Part model, mm, in its own coordinate system. A direction names the side the tool comes from. Give positions to 0.01 mm unless a question says otherwise; leave off trailing zeros. Order: outer loops, then holes, each group sorted by start corner. A loop starts at its lowest first (then second) coordinate and runs counter-clockwise, first axis right, second up. Notation, with made-up numbers: (45.25, 83.25) - (81.25, 83.25) arc R27 cw to (81.25, 113.25) - close; hole circle Ø10 at (73, 34.25). An arc over 180 degrees is marked (long way). One line per item, written item: value.
```python
from build123d import *

# Parameters (mm, degrees)
SKETCH_1_W                   = 60
SKETCH_1_H                   = 55
EXTRUDE_1_DEPTH              = 6
HOLE_WIZARD_M4_1_D           = 2.9
HOLE_WIZARD_M4_1_DEPTH       = 10
SKETCH_5_R                   = 20
CUT_EXTRUDE_1_DEPTH          = 7
SKETCH_6_W                   = 60
SKETCH_6_H                   = 55
CUT_EXTRUDE_2_DEPTH          = 7
EXTRUDE_2_DEPTH              = 6
EXTRUDE_3_DEPTH              = 6
EXTRUDE_4_DEPTH              = 4
CUT_EXTRUDE_3_DEPTH          = 11
CUT_EXTRUDE_4_DEPTH          = 6
FILLET_1_R                   = 2
EXTRUDE_5_DEPTH              = 6
CHAMFER_2_SIZE               = 5
FILLET_4_R                   = 2
CHAMFER_3_SIZE               = 1
HOLE_WIZARD_M3_2_D           = 3.3
HOLE_WIZARD_M3_2_DEPTH       = 10
HOLE_WIZARD_M3_2_CBORE_D     = 6.5
HOLE_WIZARD_M3_2_CBORE_DEPTH = 3.4
HOLE_WIZARD_M3_2_TIP         = 0.991420021


with BuildPart() as part:
    # ｽｹｯﾁ1 → ﾎﾞｽ - 押し出し1 (new body)
    with BuildSketch(Plane.XY):
        Rectangle(SKETCH_1_W, SKETCH_1_H)
    extrude(amount=EXTRUDE_1_DEPTH)

    # M4 すきま穴1
    with Locations(Plane.XY.offset(6)):
        with Locations((-20, -18), (23, 20)):
            Hole(HOLE_WIZARD_M4_1_D / 2, depth=HOLE_WIZARD_M4_1_DEPTH)

    # ｽｹｯﾁ5 → ｶｯﾄ - 押し出し1 (cut, through all)
    with BuildSketch(Plane.XY.offset(6)):
        Circle(SKETCH_5_R)
    extrude(amount=-CUT_EXTRUDE_1_DEPTH, mode=Mode.SUBTRACT)

    # ｽｹｯﾁ6 → ｶｯﾄ - 押し出し2 (cut, through all)
    with BuildSketch(Plane.XY.offset(6)):
        Rectangle(SKETCH_6_W, SKETCH_6_H)
        with BuildLine():
            ThreePointArc((-17.351208814, -20.997316342), (-22.997316342, -20.648791186), (-22.648791186, -15.002683658))
            Line((-22.648791186, -15.002683658), (-21.007829355, -13.552531342))
            ThreePointArc((-21.007829355, -13.552531342), (-16.554944912, 18.733227137), (16.03335661, 19.181539975))
            Line((16.03335661, 19.181539975), (20.351208814, 22.997316342))
            ThreePointArc((20.351208814, 22.997316342), (25.997316342, 22.648791186), (25.648791186, 17.002683658))
            Line((25.648791186, 17.002683658), (21.271672672, 13.134532414))
            ThreePointArc((21.271672672, 13.134532414), (24.04986296, 6.826718948), (25, 0))
            ThreePointArc((25, 0), (10.810307191, -22.541900062), (-15.650980674, -19.494789148))
            Line((-15.650980674, -19.494789148), (-17.351208814, -20.997316342))
        make_face(mode=Mode.SUBTRACT)
    extrude(amount=-CUT_EXTRUDE_2_DEPTH, mode=Mode.SUBTRACT)

    # ｽｹｯﾁ7 → ﾎﾞｽ - 押し出し2 (add)
    with BuildSketch(Plane.XY.offset(6)):
        with BuildLine():
            Line((0, 25), (-21.5, 25))
            Line((-21.5, 25), (-21.5, 12.757350822))
            ThreePointArc((-21.5, 12.757350822), (-12.370655388, 21.724798855), (0, 25))
        make_face()
        with BuildLine():
            ThreePointArc((-17.351208814, -20.997316342), (-18.583890076, -21.74094008), (-20, -22))
            Line((-20, -22), (-11.874342087, -22))
            ThreePointArc((-11.874342087, -22), (-13.819546614, -20.833149819), (-15.650980674, -19.494789148))
            Line((-15.650980674, -19.494789148), (-17.351208814, -20.997316342))
        make_face()
        with BuildLine():
            ThreePointArc((-21.007829355, -13.552531342), (-21.25763315, -13.157242601), (-21.5, -12.757350822))
            Line((-21.5, -12.757350822), (-21.5, -13.987472843))
            Line((-21.5, -13.987472843), (-21.007829355, -13.552531342))
        make_face()
    extrude(amount=-EXTRUDE_2_DEPTH)

    # ｽｹｯﾁ8 → ﾎﾞｽ - 押し出し3 (add)
    with BuildSketch(Plane.XY.offset(6)):
        with BuildLine():
            Line((-21.5, 12.757350822), (-21.5, 25))
            Line((-21.5, 25), (-45.717384076, -1.896129831))
            Line((-45.717384076, -1.896129831), (-23.389774269, -22))
            Line((-23.389774269, -22), (-20, -22))
            ThreePointArc((-20, -22), (-23.74094008, -19.416109924), (-22.648791186, -15.002683658))
            Line((-22.648791186, -15.002683658), (-21.5, -13.987472843))
            Line((-21.5, -13.987472843), (-21.5, -12.757350822))
            ThreePointArc((-21.5, -12.757350822), (-25, 0), (-21.5, 12.757350822))
        make_face()
    extrude(amount=-EXTRUDE_3_DEPTH)

    # ｽｹｯﾁ9 → ﾎﾞｽ - 押し出し4 (add)
    with BuildSketch(Plane(origin=(0, 0, 0), x_dir=(-1, 0, 0), z_dir=(0, 0, -1))):
        Polygon((25.649471154, -6.509032491), (32.340777217, -13.940480745), (45.717384076, -1.896129831), (39.026078012, 5.535318424), align=None)
    extrude(amount=EXTRUDE_4_DEPTH)

    # ｽｹｯﾁ10 → ｶｯﾄ - 押し出し3 (cut, through all)
    with BuildSketch(Plane(origin=(0, 0, -4), x_dir=(-1, 0, 0), z_dir=(0, 0, -1))):
        Polygon((39.026078012, 5.535318424), (21.5, 25), (13.426203622, 25), (41.258515123, -5.910913469), (45.717384076, -1.896129831), align=None)
    extrude(amount=-CUT_EXTRUDE_3_DEPTH, mode=Mode.SUBTRACT)

    # ｽｹｯﾁ12 → ｶｯﾄ - 押し出し4 (cut)
    with BuildSketch(Plane.XY.offset(6)):
        Polygon((-41.258515123, -5.910913469), (-26.47934628, -19.218136867), (-22.464562642, -14.759267914), (-37.243731485, -1.452044516), align=None)
    extrude(amount=-CUT_EXTRUDE_4_DEPTH, mode=Mode.SUBTRACT)

    # ﾌｨﾚｯﾄ1
    fillet_1_edges = [part.edges().sort_by_distance(p)[0] for p in [
        (-25.649471154, -6.509032491, -2),
        (-34.567209059, 1.520534786, -2),
        (-26.47934628, -19.218136867, 3),
    ]]
    fillet(fillet_1_edges, radius=FILLET_1_R)

    # ｽｹｯﾁ13 → ﾎﾞｽ - 押し出し5 (add)
    with BuildSketch(Plane.XY):
        Polygon((-32.340777217, -13.940480745), (-28.325993579, -9.481611793), (-37.243731485, -1.452044516), (-41.258515123, -5.910913469), align=None)
    extrude(amount=EXTRUDE_5_DEPTH)

    # 面取り2
    chamfer_2_edges = [part.edges().sort_by_distance(p)[0] for p in [
        (-36.79964617, -9.925697107, 6),
    ]]
    chamfer(chamfer_2_edges, length=CHAMFER_2_SIZE)

    # ﾌｨﾚｯﾄ4
    fillet_4_edges = [part.edges().sort_by_distance(p)[0] for p in [
        (-23.389774269, -22, 3),
        (-13.426203622, 25, 3),
        (-22.464562642, -14.759267914, 3),
        (-33.453993138, -6.20997298, 6),
        (-36.79964617, -9.925697107, 1),
        (21.271672672, 13.134532414, 3),
        (16.03335661, 19.181539975, 3),
        (-11.874342087, -22, 3),
    ]]
    fillet(fillet_4_edges, radius=FILLET_4_R)

    # 面取り3
    chamfer_3_edges = [part.edges().sort_by_distance(p)[0] for p in [
        (-29.664254792, -10.967901443, -4),
        (-32.340777217, -13.940480745, -1.914213562),
        (-36.79964617, -9.925697107, -4),
        (-38.581992697, -2.938334167, -4),
        (-30.108340106, -2.494248852, -4),
        (-34.523852534, 0.693242992, -4),
        (-26.476762948, -6.552389016, -4),
        (-24.471954461, -16.98870239, 6),
        (-24.471954461, -16.98870239, 0),
        (-24.47668202, -21.021343865, 6),
        (-25.652054486, -19.174780341, 6),
        (-25.652054486, -19.174780341, 0),
        (-24.47668202, -21.021343865, 0),
        (-25.690286025, 11.379356601, 6),
        (-28.38339591, -9.54536354, 6),
        (-26.138422936, -11.451309247, 6),
        (-17.495681538, -22, 6),
        (17.805324329, -17.549086174, 6),
        (24.071292776, 15.608615296, 6),
        (18.815379015, 21.640071403, 6),
        (7.771710455, 23.761323966, 6),
        (-13.349219538, 24.827090915, 6),
        (-23.338782098, -21.867160853, 6),
        (-17.495681538, -22, 0),
        (-26.138422936, -11.451309247, 0),
        (-24.963753087, 12.186253174, 0),
        (-6.267873126, 25, 0),
        (7.771710455, 23.761323966, 0),
        (18.815379015, 21.640071403, 0),
        (24.071292776, 15.608615296, 0),
        (17.805324329, -17.549086174, 0),
        (-13.349219538, 24.827090915, 0),
        (-23.338782098, -21.867160853, 0),
        (-41.258515123, -5.910913469, -1.914213562),
        (-39.585688607, -4.053051405, 3.5),
        (-37.870666541, -2.148326436, 5.847759065),
        (-41.156646054, -5.797776406, 0.93693974),
        (-30.667950701, -12.082618682, 3.5),
        (-28.952928635, -10.177893712, 5.847759065),
        (-32.238908148, -13.827343682, 0.93693974),
        (21.8499093, 13.07067214, 0),
        (21.8499093, 13.07067214, 6),
        (16.046656493, 19.783578925, 0),
        (16.046656493, 19.783578925, 6),
        (-11.897912356, -22.056349368, 6),
        (-11.897912356, -22.056349368, 0),
        (-23.291854436, -14.80262444, 6),
        (-23.291854436, -14.80262444, 0),
        (-20, 0, 0),
        (-20, 0, 6),
        (25.997316342, 22.648791186, 0),
        (25.997316342, 22.648791186, 6),
        (-6.267873126, 25, 6),
    ]]
    chamfer(chamfer_3_edges, length=CHAMFER_3_SIZE)

    # M3 六角穴付き頭ねじ用座ぐり穴2
    with Locations(Plane.XY.offset(6)):
        with Locations((-34.197137964, -5.540842373)):
            CounterBoreHole(HOLE_WIZARD_M3_2_D / 2, HOLE_WIZARD_M3_2_CBORE_D / 2, HOLE_WIZARD_M3_2_CBORE_DEPTH, depth=HOLE_WIZARD_M3_2_DEPTH)
            with Locations((0, 0, -(HOLE_WIZARD_M3_2_DEPTH + HOLE_WIZARD_M3_2_TIP / 2))):  # 118° drill point
                Cone(0, HOLE_WIZARD_M3_2_D / 2, HOLE_WIZARD_M3_2_TIP, mode=Mode.SUBTRACT)


solid = part.part
```
1) Pin check, flat tips, straight feed: pin 1 (2 mm diameter, centred on x = -34.2, y = -5.54, fed in from +Z); pin 2 (2 mm diameter, centred on y = -16, z = 4, fed in from +X); pin 3 (4 mm diameter, centred on x = -20, y = -18, fed in from -Z); pin 4 (5 mm diameter, centred on y = 2.5, z = 2, fed in from -X). Stop position of each tip, or through.
Outcome:
pin 1: passes through
pin 2: stops at x = 20
pin 3: stops at z = 0
pin 4: stops at x = -35.94
2) Cut at A-A, the plane z = -1.5. Give the cut face in (x, y).
Outcome:
outline: (-40.59, -5.17) - (-40.52, -6.58) - (-33.08, -13.27) - (-31.67, -13.2) - (-26.99, -8) arc R2 ccw to (-27.14, -5.17) - (-33.08, 0.18) arc R2 ccw to (-35.91, 0.03) - close; hole circle Ø3.3 at (-34.2, -5.54)
3) Which spindle directions (+Z, -Z, +X, -X, +Y, -Y) get a long thin tool onto all of the face, cutting with end or side? Do faces 4 (the cylindrical face through (-32.45, -2.8, 4.32)), 5 (the flat face through (-26.108, -11.479, 3.028)), 6 (the flat face through (-18, -22, 3)), 7 (the flat face through (-24.115, -17.329, 5.493)). Say none if no direction does.
Outcome:
face 4: +Z
face 5: +Z, -Z
face 6: +Z, -Z, -X, -Y
face 7: +Z, -X
4) Mould opens along X. For faces 1 (the flat face through (-30.777, -11.466, 3.168)), 2 (the conical face through (-25.05, -19.16, 0.4)), 3 (the flat face through (23.77, 16, 0.51)) say: released by +X, released by -X, zero draft, split by the parting line, or undercut.
Outcome:
face 1: undercut
face 2: released by -X
face 3: released by +X
5) Drill centre lines: line 1 along Y through (x, z) = (23, 2.4); line 2 along X through (y, z) = (-11.5, 1.5); line 3 along Z through (x, y) = (20, -8). Where is each one in solid material? Low to high. Write a range as from..to.
Outcome:
line 1: y = -9.8..9.8, 14.66..18.55, 21.45..24
line 2: x = -34.3..-30.14, -26.08..-16.36, 16.36..22.2
line 3: z = 0..6
